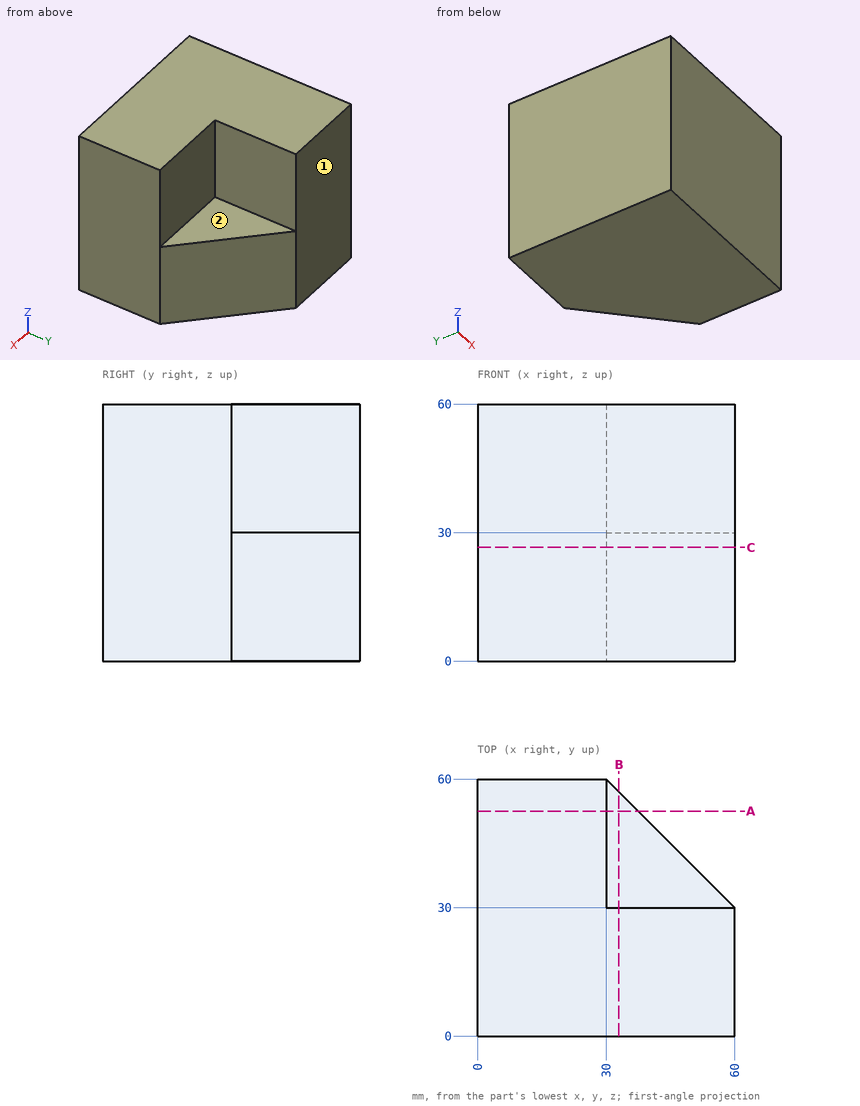
Input: dimensioned drawing with shaded views. Units: mm. Origin: part minimum x, y, z. A direction names the side the tool comes from. Give positions to 0.01 mm unless a question says otherwise; leave off trailing zeros. Order: outer loops, then holes, each group sorted by start corner. A loop starts at its lowest first (then second) coordinate and runs counter-clockwise, first axis right, second up. Notation, with made-up numbers: (78.25, 58) -> (90.25, 58) arc R22 ccw to (90.25, 70) -> close; hole circle Ø2 at (28, 86). An arc over 180 degrees is marked (long way). Answer as a JSON object with one key per item and string values.
Q1. Section C-C (z = 26.5). Output: boundary loops of the cut face in (x, y).
Entries:
{"outline": "(0, 0) -> (60, 0) -> (60, 30) -> (30, 60) -> (0, 60) -> close"}
Q2. First-contact query: pin 1 (9 mm diameter, centred on x = 49.5, z = 39.5, fed in from +Y); pin 2 (1 mm diameter, centred on y = 45, z = 22, fed in from -X); pin 3 (15 mm diameter, centred on x = 38.5, y = 41, fed in from +Z); pin 4 (1.5 mm diameter, centred on y = 35.5, z = 34, fed in from +X). Flat tips, straight axial feed; report the tip coordinate or a pass-through.
Entries:
{"pin 1": "stops at y = 30", "pin 2": "stops at x = 0", "pin 3": "stops at z = 30", "pin 4": "stops at x = 30"}
Q3. Section B-B (x = 33). Output: boundary loops of the cut face in (y, z), plus the area to 3 significant figures.
Entries:
{"outline": "(0, 0) -> (57, 0) -> (57, 30) -> (30, 30) -> (30, 60) -> (0, 60) -> close", "area": "2,610 mm^2"}
Q4. Section A-A (y = 52.5). Output: boundary loops of the cut face in (x, z), plus the area to 4 significant figures.
Entries:
{"outline": "(0, 0) -> (37.5, 0) -> (37.5, 30) -> (30, 30) -> (30, 60) -> (0, 60) -> close", "area": "2,025 mm^2"}
Q5. Access query for the marked faces 1 and 2. Directions: +Z, -Z, +X, -X, +Y, -Y. A direction counts if a zero-diameter tool reaches every point of the face in a straight line with its end or side. Return the directions, or none.
Entries:
{"face 1": "+Z, -Z, +X, -X, +Y", "face 2": "+Z, +X, +Y"}
Q6. Material intervals for probe 1 along X at (y, z) = (35, 49); probe 2 along Y at (x, z) = (42, 3.5), sorted ascending.
Entries:
{"probe 1": "x = 0 to 30", "probe 2": "y = 0 to 48"}
